from build123d import *

# Parameters (mm, degrees)
BOSS_EXTRUDE4_DEPTH                                 = 180.34
CBORE_FOR_4_BINDING_HEAD_MACHINE_SCREW1_D           = 3.2639
CBORE_FOR_4_BINDING_HEAD_MACHINE_SCREW1_CBORE_D     = 6.74624
CBORE_FOR_4_BINDING_HEAD_MACHINE_SCREW1_CBORE_DEPTH = 1.7272
FILLET1_R                                           = 1.27
CBORE_FOR_4_BINDING_HEAD_MACHINE_SCREW2_D           = 3.2639
CBORE_FOR_4_BINDING_HEAD_MACHINE_SCREW2_CBORE_D     = 6.74624
CBORE_FOR_4_BINDING_HEAD_MACHINE_SCREW2_CBORE_DEPTH = 1.7272


with BuildPart() as part:
    # Sketch5 → Boss-Extrude4 (new body)
    with BuildSketch(Plane(origin=(0, 0, 0), x_dir=(1, 0, 0), z_dir=(0, 1, 0))):
        with BuildLine():
            Line((0, 0), (15.9512, 0))
            Line((15.9512, 0), (13.9573, -6.35))
            ThreePointArc((13.9573, -6.35), (7.9756, -6.438062229), (1.9939, -6.35))
            Line((1.9939, -6.35), (0, 0))
        make_face()
    extrude(amount=BOSS_EXTRUDE4_DEPTH)

    # CBORE for #4 Binding Head Machine Screw1 (through all)
    with Locations(Plane(origin=(0, 0, 0), x_dir=(-1, 0, 0), z_dir=(0, 0, -1))):
        with Locations((-7.827128231, 133.35), (-7.827128231, 12.7)):
            CounterBoreHole(CBORE_FOR_4_BINDING_HEAD_MACHINE_SCREW1_D / 2, CBORE_FOR_4_BINDING_HEAD_MACHINE_SCREW1_CBORE_D / 2, CBORE_FOR_4_BINDING_HEAD_MACHINE_SCREW1_CBORE_DEPTH)

    # Fillet1
    fillet1_edges = [part.edges().sort_by_distance(p)[0] for p in [
        (0, 90.17, 0),
        (15.9512, 90.17, 0),
    ]]
    fillet(fillet1_edges, radius=FILLET1_R)

    # CBORE for #4 Binding Head Machine Screw2 (through all)
    with Locations(Plane(origin=(7.9756, 152.424464219, 6.438062229), x_dir=(1, 0, 0), z_dir=(0, 0, 1))):
        with Locations((0, 0)):
            CounterBoreHole(CBORE_FOR_4_BINDING_HEAD_MACHINE_SCREW2_D / 2, CBORE_FOR_4_BINDING_HEAD_MACHINE_SCREW2_CBORE_D / 2, CBORE_FOR_4_BINDING_HEAD_MACHINE_SCREW2_CBORE_DEPTH)


solid = part.part
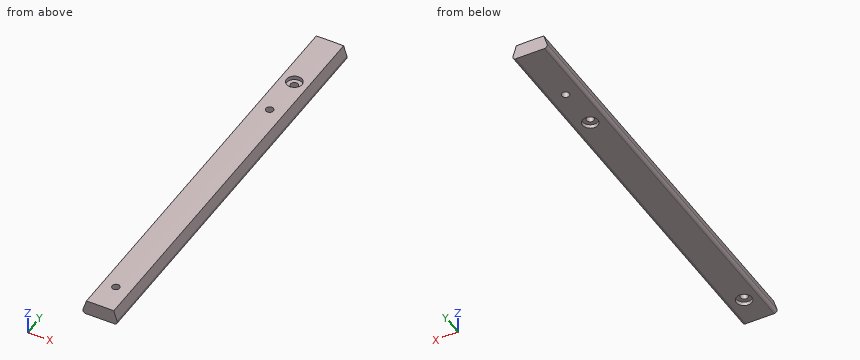
Verification items for the finished model (mm, model axes). Coordinates: 2 decimals unless noted, no trailing zeros. Order: outer loops, then holes, each group sorted by start corner. A loop starts at its lowest first (then second) coordinate and runs counter-clockwise, first axis right, second up. Notation, with made-up numbers: (-26.75, 62) -> (-15.75, 62) arc R10 cw to (-15.75, 78) -> close; hole circle Ø4 at (1.25, -21.5). An arc over 180 degrees is marked (long way). Use CSV: the item, a comma, the result in double quotes. Start each with the question number.
Q1. Depth check by flat-ended pin: P1, Ø2, axis at x = 6, y = 93.5, coming from the +Z side; P2, Ø2, axis at x = 7.5, y = 12.5, coming from the -Z side; P3, Ø3, axis at y = 116, z = 5, coming from the -X side; P4, Ø2, axis at x = 7, y = 151, coming from the +Z side. Enter the tip coordinate at first touch or a pass-through.
Q2. Section check A-A, the plane y = 12.7. Record the cut outline in (x, z), and give its area (3 significant figures).
Q3. Section check B-B, the plane y = 50.5. Record the cut outline in (x, z).
Q4. Thickness scan on line 1 along Y through (x, z) = (10, 0.75); line 2 along Y through (x, z) = (8.25, 5.75); line 3 along X through (y, z) = (38.5, 6.25). Record the ranges inside material, lowest first.
Returned:
1,P1,"stops at z = 6.44"
1,P2,"passes through"
1,P3,"stops at x = 1.1"
1,P4,"stops at z = 4.71"
2,outline,"(0.52, 1.65) arc R1.27 ccw to (1.73, 0) -> (4.45, 0) -> (4.45, 1.73) -> (6.2, 1.73) -> (6.2, 6.43) arc R203.2 ccw to (1.99, 6.35) -> close; (9.46, 1.73) -> (11.2, 1.73) -> (11.2, 0) -> (14.22, 0) arc R1.27 ccw to (15.43, 1.65) -> (13.96, 6.35) arc R203.2 ccw to (9.46, 6.43) -> close"
2,area,"60.9 mm^2"
3,outline,"(0.52, 1.65) arc R1.27 ccw to (1.73, 0) -> (14.22, 0) arc R1.27 ccw to (15.43, 1.65) -> (13.96, 6.35) arc R203.2 ccw to (1.99, 6.35) -> close"
4,line 1,"y = 0 to 10.12, 15.28 to 130.77, 135.93 to 180.34"
4,line 2,"y = 0 to 11.12, 14.28 to 131.77, 134.93 to 149.06, 155.79 to 180.34"
4,line 3,"x = 1.96 to 13.99"
